Verification items for the finished model (mm, model axes). A direction names the side the tool comes from. Round coordinates to 2 decimals unless told otherwise and drop trailing zeros. Write each loop counter-clockwise with the first axis right and the second up, starting at its lowest first coordinate (ties: lowest second). Pieces come first, ordered by that corner, then holes. Notation, with made-up numbers: (72.25, 35.25) - (79.25, 35.25) arc R6 ccw to (79.25, 41.25) - close; hole circle Ø3 at (11.25, 66). An arc over 180 degrees is marked (long way). Answer as a JSON object with one key per item and string values.
Autodesk Inventor part; units mm, degrees
ref_plane "YZ Plane" through (0, 0, 0) normal (1, 0, 0) x (0, 1, 0)
ref_plane "XZ Plane" through (0, 0, 0) normal (0, 1, 0) x (-1, 0, 0)
ref_plane "XY Plane" through (0, 0, 0) normal (0, 0, 1) x (1, 0, 0)
sketch "Skizze1" plane through (0, 0, 0) normal (0, 0, 1) x (1, 0, 0)
  point P0 (0, 0)
sketch "Skizze2" plane through (0, 0, 0) normal (0, 0, 1) x (1, 0, 0)
  line L0 (-15.5739, -1.2028) -> (16.4261, -1.2028)
  line L1 (16.4261, -1.2028) -> (16.4261, -10.2028)
  line L2 (16.4261, -10.2028) -> (-15.5739, -10.2028)
  line L3 (-15.5739, -10.2028) -> (-15.5739, -1.2028)
  point P0 (0, 0)
  dimension "d0" = 32
  dimension "d1" = 9
extrude "Extrusion1" add sketch "Skizze2" along normal blind 10.5
sketch "Skizze3" plane through (16.4261, -10.2028, 0) normal (1, 0, 0) x (0, 0, -1)
  point P0 (0, 10.2028)
sketch "Skizze4" plane through (-15.5739, -1.2028, 0) normal (0, 1, 0) x (1, 0, 0)
  line L0 (0, 0) -> (0, -10.5)
  line L1 (0, 0) -> (32, 0)
  point P0 (15.5739, 0)
  point P1 (16, -5.25)
  point P2 (7.496, -5.25)
  point P3 (24.504, -5.25)
  dimension "d4" = 8.504
  dimension "d5" = 8.504
  dimension "d6" = 16
  dimension "d14" = 5.25
  dimension "d15" = 5.25
sketch "Skizze5" plane through (0, 0, 0) normal (0, 0, -1) x (-1, 0, 0)
  point P0 (0, 0)
sketch "Skizze6" plane through (0, 0, 0) normal (0, 0, -1) x (-1, 0, 0)
  line L0 (-4.8511, -7.7528) -> (3.9989, -7.7528)
  line L1 (3.9989, -7.7528) -> (3.9989, -3.6528)
  line L2 (3.9989, -3.6528) -> (-4.8511, -3.6528)
  line L3 (-4.8511, -3.6528) -> (-4.8511, -7.7528)
  line L4 (-16.4261, -10.2028) -> (15.5739, -10.2028)
  line L5 (15.5739, -10.2028) -> (15.5739, -1.2028)
  point P0 (0, 0)
  dimension "d16" = 8.85
  dimension "d17" = 4.1
  dimension "d18" = 2.45
  dimension "d19" = 11.575
extrude "Extrusion2" cut sketch "Skizze6" against normal blind 9.3
sketch "Skizze7" plane through (-15.5739, -10.2028, 0) normal (0, -1, 0) x (1, 0, 0)
  point P0 (15.5739, 0)
sketch "Skizze8" plane through (0, 0, 0) normal (0, 0, -1) x (-1, 0, 0)
  point P0 (0, 0)
sketch "Skizze9" plane through (-15.5739, -10.2028, 0) normal (0, -1, 0) x (1, 0, 0)
  line L0 (0, 0) -> (32, 0)
  line L1 (4.9045, 0) -> (9.9045, 0)
  line L2 (9.9045, 0) -> (9.9045, 1.2)
  line L3 (9.9045, 1.2) -> (4.9045, 1.2)
  line L4 (4.9045, 1.2) -> (4.9045, 0)
  point P0 (15.5739, 0)
  dimension "d22" = 1.2
  dimension "d23" = 5
extrude "Extrusion3" add sketch "Skizze9" along normal blind 15
sketch "Skizze10" plane through (0, 0, 0) normal (0, 0, -1) x (-1, 0, 0)
  line L0 (5.6694, -25.2028) -> (10.6694, -25.2028)
  line L1 (15.5739, -1.2028) -> (-16.4261, -1.2028)
  line L2 (10.6694, -25.2028) -> (5.6694, -25.2028)
  line L3 (5.6694, -25.2028) -> (5.6694, -1.2028)
  line L4 (5.6694, -1.2028) -> (10.6694, -1.2028)
  line L5 (10.6694, -1.2028) -> (10.6694, -25.2028)
  point P0 (0, 0)
  dimension "d26" = 5
extrude "Extrusion4" add sketch "Skizze10" along normal blind 5
sketch "Skizze11" plane through (-15.5739, -25.2028, 0) normal (0, -1, 0) x (1, 0, 0)
  line L0 (4.9045, -5) -> (9.9045, -5)
  line L1 (6.7795, -5) -> (8.0295, -5)
  line L2 (8.0295, -5) -> (8.0295, -0.9525)
  line L3 (8.0295, -0.9525) -> (6.7795, -0.9525)
  line L4 (6.7795, -0.9525) -> (6.7795, -5)
  line L5 (9.9045, 1.2) -> (9.9045, -5)
  point P0 (15.5739, 0)
  dimension "d29" = 1.25
  dimension "d30" = 1.875
  dimension "d31" = 4.0475
extrude "Extrusion5" cut sketch "Skizze11" against normal blind 22
sketch "Skizze12" plane through (-15.5739, -25.2028, 0) normal (0, -1, 0) x (1, 0, 0)
  line L0 (9.9045, 1.2) -> (9.9045, 0)
  line L1 (4.9045, 0) -> (4.9045, 1.2)
  line L2 (9.9045, 1.2) -> (4.9045, 1.2)
  line L3 (4.9045, 1.2) -> (4.9045, 0)
  line L4 (4.9045, 0) -> (9.9045, 0)
  line L5 (9.9045, 0) -> (9.9045, 1.2)
  point P0 (15.5739, 0)
extrude "Extrusion6" cut sketch "Skizze12" against normal blind 15
sketch "Skizze13" plane through (0, 0, 0) normal (0, 1, 0) x (-1, 0, 0)
  line L0 (5.6694, 0) -> (-16.4261, 0)
  line L1 (-6.5211, 0) -> (-11.5211, 0)
  line L2 (-11.5211, 0) -> (-11.5211, -5)
  line L3 (-11.5211, -5) -> (-6.5211, -5)
  line L4 (-6.5211, -5) -> (-6.5211, 0)
  line L5 (-16.4261, 0) -> (-16.4261, 10.5)
  point P0 (0, 0)
  dimension "d36" = 5
  dimension "d37" = 5
  dimension "d38" = 4.905
extrude "Extrusion7" add sketch "Skizze13" against normal blind 25.203
sketch "Skizze14" plane through (6.5211, 0, 0) normal (0, 0, 1) x (1, 0, 0)
  line L0 (5, -1.2028) -> (9.905, -1.2028)
  line L1 (0, 0) -> (0, -25.203)
  line L2 (5, -1.2028) -> (0, -1.2028)
  line L3 (0, -1.2028) -> (0, 0)
  line L4 (0, 0) -> (5, 0)
  line L5 (5, 0) -> (5, -1.2028)
  point P0 (-6.5211, 0)
extrude "Extrusion8" cut sketch "Skizze14" against normal blind 25
sketch "Skizze15" plane through (0, -25.203, 0) normal (0, -1, 0) x (1, 0, 0)
  line L0 (6.5211, -5) -> (11.5211, -5)
  line L1 (8.3961, -5) -> (9.6461, -5)
  line L2 (9.6461, -5) -> (9.6461, -0.952)
  line L3 (9.6461, -0.952) -> (8.3961, -0.952)
  line L4 (8.3961, -0.952) -> (8.3961, -5)
  line L5 (11.5211, -5) -> (11.5211, 0)
  point P0 (0, 0)
  dimension "d43" = 1.25
  dimension "d44" = 4.048
  dimension "d45" = 1.875
extrude "Extrusion9" cut sketch "Skizze15" against normal blind 22
sketch "Skizze16" plane through (-15.5739, -25.2028, 0) normal (0, -1, 0) x (1, 0, 0)
  line L0 (0, 0) -> (4.9045, 0)
  line L1 (4.9045, -5) -> (9.9045, -5)
  line L2 (4.9045, 0) -> (9.9045, 0)
  line L3 (9.9045, 0) -> (9.9045, -5)
  line L4 (9.9045, -5) -> (4.9045, -5)
  line L5 (4.9045, -5) -> (4.9045, 0)
  point P0 (15.5739, 0)
extrude "Extrusion10" cut sketch "Skizze16" against normal blind 25
hole "Bohrung2" at (0.4261, -1.2028, 5.25) direction (0, -1, 0) diameter 6 end through all
hole "Bohrung3" at (-8.0779, -1.2028, 5.25) at (8.9301, -1.2028, 5.25) direction (0, -1, 0) diameter 6.5 end through all
properties part number "Objektträgerhalter 2afinal"
1. Mould release check, pull along Y, two halves, no side actions. Record for faces 5 (the face through (-3.999, -6, 5)), 6 (the face through (8, -25.203, -2)), 7 (the face through (6.521, -13, -3)): released by +Y, released by -Y, zero draft, split by the parting line, or undercut.
Completed:
{"face 5": "undercut", "face 6": "released by -Y", "face 7": "zero draft"}
2. Cross-section at D-D (x = 4). Record the boundary of the cut face in (y, z), plus the area to 3 significant figures.
Completed:
{"outline": "(-10.2, 0) - (-7.75, 0) - (-7.75, 9.3) - (-3.65, 9.3) - (-3.65, 0) - (-1.2, 0) - (-1.2, 10.5) - (-10.2, 10.5) - close", "area": "56.4 mm^2"}
3. Go/stop test with flat-tipped pins: pin 1 (6 mm diameter, centred on x = -3.5, y = -8, fed in from -Z); pin 2 (5.5 mm diameter, centred on y = -9, z = -3.5, fed in from -X); pin 3 (4.5 mm diameter, centred on y = -12.5, z = -2.5, fed in from +X). Record where each tip stops, or that it passes through.
Completed:
{"pin 1": "stops at z = 0", "pin 2": "stops at x = 6.52", "pin 3": "stops at x = 11.52"}
4. Cross-section at C-C (y = -13.5). Record the boundary of the cut face in (x, z).
Completed:
{"outline": "(6.52, -5) - (8.4, -5) - (8.4, -0.95) - (9.65, -0.95) - (9.65, -5) - (11.52, -5) - (11.52, 0) - (6.52, 0) - close"}
5. Access from +Z, -Z, +X, -X, +Y, -Y to the whole of each face (thin tool, end or side, straight path). Record for faces 1 (the face through (9, -18, 0)), 2 (the face through (4.851, -6, 5)), 3 (the face through (9.646, -14, -3)), 4 (the face through (14, -6, 0)).
Completed:
{"face 1": "+Z, +X, -X, -Y", "face 2": "-Z", "face 3": "-Z, -Y", "face 4": "-Z, +X, +Y, -Y"}
6. Cross-section at B-B (x = -6.5). Record the boundary of the cut face in (y, z).
Completed:
{"outline": "(-10.2, 0) - (-1.2, 0) - (-1.2, 2.41) - (-10.2, 2.41) - close; (-10.2, 8.09) - (-1.2, 8.09) - (-1.2, 10.5) - (-10.2, 10.5) - close"}
7. Material ranges on probe 1 along X at (y, z) = (-1.85, 5.25); probe 2 along X at (y, z) = (-15.75, -2.5); probe 3 along Y at (x, z) = (-3, 4), recorded low to high. Write a range as from..to.
Completed:
{"probe 1": "x = -15.57..-11.33, -4.83..-2.57, 3.43..5.68, 12.18..16.43", "probe 2": "x = 6.52..8.4, 9.65..11.52", "probe 3": "y = -10.2..-7.75, -3.65..-1.2"}
8. Cross-section at A-A (z = 5.25). Record the boundary of the cut face in (x, y).
Completed:
{"outline": "(-15.57, -10.2) - (-11.33, -10.2) - (-11.33, -1.2) - (-15.57, -1.2) - close; (-4.83, -10.2) - (-2.57, -10.2) - (-2.57, -7.75) - (-4, -7.75) - (-4, -3.65) - (-2.57, -3.65) - (-2.57, -1.2) - (-4.83, -1.2) - close; (3.43, -10.2) - (5.68, -10.2) - (5.68, -1.2) - (3.43, -1.2) - (3.43, -3.65) - (4.85, -3.65) - (4.85, -7.75) - (3.43, -7.75) - close; (12.18, -10.2) - (16.43, -10.2) - (16.43, -1.2) - (12.18, -1.2) - close"}
